Autodesk Inventor part; units mm, degrees
ref_plane "工作平面1" through (0, 0, -40) normal (0, 0, -1) x (-1, 0, 0)
ref_plane "工作平面2" through (0, -19.075, 0) normal (0, 0, 1) x (1, 0, 0)
ref_plane "工作平面3" through (-19.075, 0, 5) normal (0, 0, 1) x (1, 0, 0)
ref_plane "工作平面1" through (0, 0, -40) normal (0, 0, -1) x (-1, 0, 0)
sketch "草圖1" plane through (0, 0, -40) normal (0, 0, -1) x (-1, 0, 0)
  line L0 (-15.075, 14.075) -> (-15.075, 19.075)
  line L1 (-19.075, 19.075) -> (-15.075, 19.075)
  line L2 (-19.075, 14.075) -> (-19.075, 19.075)
  line L3 (-15.075, 14.075) -> (-19.075, 14.075)
  line L4 (-15.075, -19.075) -> (-15.075, -14.075)
  line L5 (-19.075, -14.075) -> (-15.075, -14.075)
  line L6 (-19.075, -19.075) -> (-19.075, -14.075)
  line L7 (-15.075, -19.075) -> (-19.075, -19.075)
  line L8 (-19.075, 14.075) -> (-19.075, -14.075)
  line L9 (-15.075, -14.075) -> (-15.075, 14.075)
  point P0 (0, 0)
extrude "擠出1" add sketch "草圖1" along normal blind 5
sketch "草圖2" plane through (0, 0, -40) normal (0, 0, 1) x (1, 0, 0)
  line L0 (15.075, -19.075) -> (15.075, 19.075)
  line L1 (19.075, -19.075) -> (15.075, -19.075)
  line L2 (19.075, 19.075) -> (19.075, -19.075)
  line L3 (15.075, 19.075) -> (19.075, 19.075)
  line L4 (0, 14.075) -> (19.075, 14.075)
  line L5 (19.075, -14.075) -> (0, -14.075)
  point P0 (0, 0)
  point P1 (15.075, -14.075)
  point P2 (15.075, 14.075)
ref_plane "工作平面2" through (0, -19.075, 0) normal (0, 0, 1) x (1, 0, 0)
extrude "擠出2" add sketch "草圖2" along normal up to surface (40 mm away) contours L0 L4 L2 L5
sketch "草圖3" plane through (15.075, -14.075, 0) normal (0, 0, 1) x (1, 0, 0)
  line L0 (-15.075, 33.15) -> (-15.075, 28.15)
  line L1 (-15.075, 28.15) -> (4, 28.15)
  line L2 (4, 28.15) -> (4, 33.15)
  line L3 (4, 33.15) -> (-15.075, 33.15)
  line L4 (4, 0) -> (0, 0)
  line L5 (4, 28.15) -> (4, 0)
  line L6 (0, 28.15) -> (4, 28.15)
  line L7 (0, 0) -> (0, 28.15)
  line L8 (-15.075, 0) -> (-15.075, -5)
  line L9 (-15.075, -5) -> (4, -5)
  line L10 (4, -5) -> (4, 0)
  line L11 (4, 0) -> (-15.075, 0)
  point P0 (-15.075, 14.075)
  point P1 (0, 28.15)
  point P2 (4, 28.15)
ref_plane "工作平面3" through (-19.075, 0, 5) normal (0, 0, 1) x (1, 0, 0)
extrude "擠出3" add sketch "草圖3" along normal up to surface (5 mm away)
sketch "草圖4" plane through (0, -19.075, 5) normal (0, 0, 1) x (1, 0, 0)
  arc A0 (0, 38.15) -> (0, 0) centre (0, 19.075) ccw
  circle A1 centre (0, 19.075) radius 19.075
  arc A2 (0, 36.65) -> (0, 1.5) centre (0, 19.075) ccw
  circle A3 centre (0, 19.075) radius 17.575
  line L0 (0, 38.15) -> (0, 33.15)
  line L1 (0, 38.15) -> (0, 0)
  point P0 (0, 1.5)
  point P1 (0, 38.15)
  point P2 (0, 1.5)
  point P3 (0, 38.15)
extrude "擠出4" add sketch "草圖4" along normal blind 1 contours A1 L1 A3 L0
sketch "草圖5" plane through (15.075, -14.075, 0) normal (0, 0, -1) x (-1, 0, 0)
  arc A0 (15.075, 0) -> (15.075, 28.15) centre (15.075, 14.075) ccw
  circle A1 centre (15.075, 14.075) radius 14.075
  line L0 (15.075, 28.15) -> (-4, 28.15)
  line L1 (0, -5) -> (0, 33.15)
  line L2 (-4, 0) -> (15.075, 0)
  point P0 (0, 0)
  point P1 (15.075, 28.15)
  point P2 (0, 28.15)
extrude "擠出5" add sketch "草圖5" against normal up to surface (5 mm away) contours L2 L1 L0 A1
sketch "草圖6" plane through (0, 0, 5) normal (0, 0, 1) x (1, 0, 0)
  arc A0 (0, -17.575) -> (0, 17.575) centre (0, 0) ccw
  line L0 (0, 14.075) -> (0, 17.575)
  arc A1 (0, -14.075) -> (0, 14.075) centre (0, 0) ccw
  line L1 (0, -17.575) -> (0, -14.075)
ref_plane "工作平面4" through (-14.075, -17.575, 27.5) normal (0, 0, -1) x (0, 1, 0)
extrude "擠出6" add sketch "草圖6" along normal up to surface (22.5 mm away)
sketch "草圖7" plane through (0, 0, 27.5) normal (0, 0, 1) x (1, 0, 0)
  line L0 (17.223, -3.5) -> (7.746, -3.5)
  arc A0 (7.746, 3.5) -> (7.746, -3.5) centre (0, 0) ccw
  line L1 (7.746, 3.5) -> (17.223, 3.5)
  arc A1 (17.223, 3.5) -> (17.223, -3.5) centre (0, 0) ccw
  circle A2 centre (7.7782, 7.7782) radius 1.6
  circle A3 centre (-7.7782, 7.7782) radius 1.6
  circle A4 centre (7.7782, -7.7782) radius 1.6
  circle A5 centre (-7.7782, -7.7782) radius 1.6
  arc A6 (0, -17.575) -> (0, 17.575) centre (0, 0) ccw
  circle A7 centre (0, 0) radius 8.5
  point P0 (7.746, -3.5)
  point P1 (7.746, 3.5)
ref_plane "工作平面5" through (-17.575, -17.575, 32.5) normal (0, 0, 1) x (1, 0, 0)
extrude "擠出7" add sketch "草圖7" along normal up to surface (5 mm away) contours L0 A7 L1 A6
sketch "草圖8" plane through (15.075, -19.075, -45) normal (-1, 0, 0) x (0, 0, 1)
  line L0 (45, 5) -> (45, 33.15)
  line L1 (5, 33.15) -> (45, 33.15)
  line L2 (5, 33.15) -> (5, 38.15)
  line L3 (5, 38.15) -> (0, 38.15)
  line L4 (0, 0) -> (0, 38.15)
  line L5 (5, 0) -> (0, 0)
  line L6 (5, 0) -> (5, 5)
  line L7 (5, 5) -> (45, 5)
  point P0 (45, 19.075)
extrude "擠出8" add sketch "草圖8" along normal blind 1
sketch "草圖9" plane through (0, 0, -45) normal (0, 0, -1) x (-1, 0, 0)
  line L0 (-19.075, 19.075) -> (-14.075, 19.075)
  line L1 (-19.075, 19.075) -> (-19.075, -19.075)
  line L2 (-19.075, -19.075) -> (-14.075, -19.075)
  line L3 (-14.075, 19.075) -> (-14.075, -19.075)
  point P0 (0, 0)
extrude "擠出9" cut sketch "草圖9" against normal blind 16.5
properties part number "j4 motor mount cover_3D 列印"
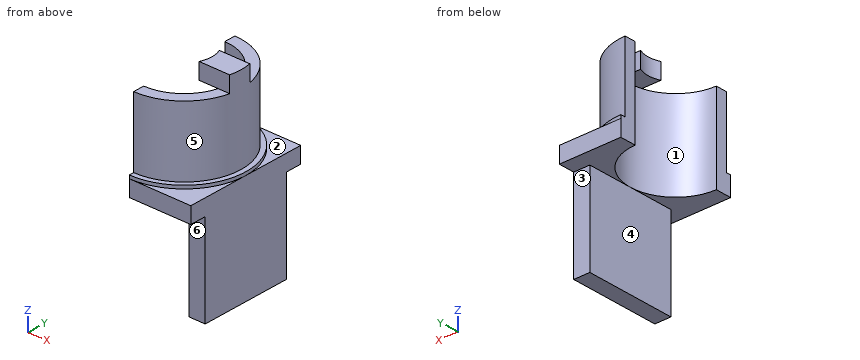
Can you work these out from the model? Positions are in its coordinate system, mm. Face numbers are marked on the shaded views. A direction names the side the tool comes from. Round coordinates to 2 decimals unless told otherwise and drop trailing zeros. Loops run counter-clockwise (first coordinate to the right, second up) from the corner with the lowest first, then second, coordinate; pieces in that order, holes last. Notation, with made-up numbers: (-31.75, 19) -> (-0.75, 19) arc R24 cw to (-0.75, 50) -> close; hole circle Ø3 at (-34, 4.5). An arc over 180 degrees is marked (long way). One line per item, written item: value. Start each with the question number.
1. If I drill on probe 1 along Z at (x, y) = (13.25, 11); probe 2 along Y at (x, z) = (18.25, -4.5) (3 decimals); probe 3 along Y at (x, z) = (9, 0.5) (3 decimals), over which ranges is the centre line in solid material (lowest first)?
2. If we section it at B-B, the plane y = -7: Write out the boundary of the cut face in (x, z) (3 decimals), then the cut area to 3 significant figures.
3. If we section it at C-C, the plane z = 10.5: Write out the boundary of the cut face in (x, y) (3 decimals), then the cut area to 3 significant figures.
4. If we section it at D-D, the plane x = 15: Write out the boundary of the cut face in (y, z) (3 decimals), then the cut area to 3 significant figures.
5. For pin 1 (1.5 mm diameter, centred on x = 13.5, z = 30, fed in from -Y); pin 2 (2 mm diameter, centred on x = 12, z = 22, fed in from -Y); pin 3 (4 mm diameter, centred on x = 16, z = -9.5, fed in from -Y) (3 decimals), each with a flat end and sliding along its axis, tell me the tip position at first contact or that it passes through.
6. If we mould it in two halves opening along Y, with no side actions, what happens to the marked faces 1, 2 and 3? For each: pulls with the +Y half, pulls with the -Y half, needs draft (parallel to the pull), parting line crosses it, or undercut.
7. For the marked faces 4, 5 and 6, which set-ups out of +Z, -Z, +X, -X, +Y, -Y let a thin tool reach every point of the face, with its end or its side?
8. If we section it at A-A, the plane x = 2.5: Write out the boundary of the cut face in (y, z) (3 decimals), then the cut area to 3 significant figures.
Calculated:
1. probe 1: z = 0 to 27.5
1. probe 2: y = -14.075 to 14.075
1. probe 3: y = -19.075 to -10.822, 10.822 to 19.075
2. outline: (12.211, 0) -> (14.075, 0) -> (14.075, -28.5) -> (19.075, -28.5) -> (19.075, 5) -> (17.744, 5) -> (17.744, 6) -> (16.121, 6) -> (16.121, 27.5) -> (12.211, 27.5) -> close
2. area: 266 mm²
3. outline: (0, -17.575) arc R17.575 ccw to (0, 17.575) -> (0, 14.075) arc R14.075 cw to (0, -14.075) -> close
3. area: 174 mm²
4. outline: (-19.075, 0) -> (-14.075, 0) -> (-14.075, -28.5) -> (14.075, -28.5) -> (14.075, 0) -> (19.075, 0) -> (19.075, 5) -> (11.784, 5) -> (11.784, 6) -> (9.159, 6) -> (9.159, 27.5) -> (3.5, 27.5) -> (3.5, 32.5) -> (-3.5, 32.5) -> (-3.5, 27.5) -> (-9.159, 27.5) -> (-9.159, 6) -> (-11.784, 6) -> (-11.784, 5) -> (-19.075, 5) -> close
4. area: 1,450 mm²
5. pin 1: stops at y = -3.5
5. pin 2: stops at y = -13.71
5. pin 3: stops at y = -14.075
6. face 1: undercut
6. face 2: needs draft
6. face 3: pulls with the +Y half
7. face 4: -Z, -X, +Y, -Y
7. face 5: +Z, +X
7. face 6: -Z, +X, -X, -Y
8. outline: (-19.075, 0) -> (-13.851, 0) -> (-13.851, 27.5) -> (-17.396, 27.5) -> (-17.396, 6) -> (-18.91, 6) -> (-18.91, 5) -> (-19.075, 5) -> close; (13.851, 0) -> (19.075, 0) -> (19.075, 5) -> (18.91, 5) -> (18.91, 6) -> (17.396, 6) -> (17.396, 27.5) -> (13.851, 27.5) -> close
8. area: 215 mm²
